Could you check a few things on this model? Use its own coordinates, in mm. Give positions to 0.01 mm unless a question says otherwise; leave off trailing zeros. Order: outer loops, then holes, each group sorted by start corner. A loop starts at its lowest first (then second) coordinate and runs counter-clockwise, first axis right, second up. Notation, with made-up numbers: M -27,-2.75 L 6,-2.75 A29 ccw 6,31.25 Z; hole C 31,15 d1. An arc over 180 degrees is marked long. Return JSON: item names as keys, results as strings. Group by question number.
```python
from build123d import *

# Parameters (mm, degrees)
SKIZZE1_W                       = 30
SKIZZE1_H                       = 15
SKIZZE1_R                       = 2.1
AUFSATZ_LINEAR_AUSTRAGEN1_DEPTH = 2


with BuildPart() as part:
    # Skizze1 → Aufsatz-Linear austragen1 (new body, symmetric)
    with BuildSketch(Plane(origin=(0, 0, 0), x_dir=(1, 0, 0), z_dir=(0, 1, 0))):
        Rectangle(SKIZZE1_W, SKIZZE1_H)
        Circle(SKIZZE1_R, mode=Mode.SUBTRACT)
    extrude(amount=AUFSATZ_LINEAR_AUSTRAGEN1_DEPTH, both=True)


solid = part.part
```
1. If we mould it in two halves opening along Z, with no side actions, what happens to faces 1 (the cylindrical face through (2.003, -0.028, -0.631)), 2 (the flat face through (0, 0, 7.5)), 3 (the flat face through (15, 0, 0)), 4 (the flat face through (0, 0, -7.5))? For each: pulls with the +Z half, pulls with the -Z half, needs draft (parallel to the pull), parting line crosses it, or undercut.
2. Imagine slicing it at B-B, the plane z = 0. Please give me the cut outline in (x, y).
3. Imagine slicing it at C-C, the plane y = 1.25. Please give me the cut outline in (x, z), plus the area to 3 significant figures.
4. Imagine slicing it at A-A, the plane x = 0. Please give me the cut outline in (y, z), plus the area to 3 significant figures.
5. I need wall thicknesses on L1, parallel to X at y = -0.2, z = 0; L2, parallel to Z at x = 0, y = -1.05; L3, parallel to X at y = 0.9, z = 1.25. Which ranges of each line are inside material? Lowest first, please. Write a range as from..to.
Values:
{
 "1": {"face 1": "undercut", "face 2": "pulls with the +Z half", "face 3": "needs draft", "face 4": "pulls with the -Z half"},
 "2": {"outline": "M -15,-2 L -2.1,-2 L -2.1,2 L -15,2 Z; M 2.1,-2 L 15,-2 L 15,2 L 2.1,2 Z"},
 "3": {"outline": "M -15,-7.5 L 15,-7.5 L 15,7.5 L -15,7.5 Z; hole C 0,0 d4.2", "area": "436 mm²"},
 "4": {"outline": "M -2,-7.5 L 2,-7.5 L 2,-2.1 L -2,-2.1 Z; M -2,2.1 L 2,2.1 L 2,7.5 L -2,7.5 Z", "area": "43.2 mm²"},
 "5": {"L1": "x = -15..-2.1, 2.1..15", "L2": "z = -7.5..-2.1, 2.1..7.5", "L3": "x = -15..-1.69, 1.69..15"}
}
